```python
from build123d import *

# Parameters (mm, degrees)
SKETCH2_W           = 219.075
SKETCH2_H           = 241.3
BOSS_EXTRUDE1_DEPTH = 3.175
SKETCH3_W           = 3.175
SKETCH3_H           = 76.2
SKETCH3_W_2         = 76.2
SKETCH3_H_2         = 3.175
CUT_EXTRUDE1_DEPTH  = 4.175
SKETCH4_W           = 12.7
SKETCH4_H           = 20.32
SKETCH4_H_2         = 12.7
CUT_EXTRUDE2_DEPTH  = 4.175


with BuildPart() as part:
    # Sketch2 → Boss-Extrude1 (new body)
    with BuildSketch(Plane(origin=(0, 0, 0), x_dir=(1, 0, 0), z_dir=(0, 1, 0))):
        with Locations((109.5375, 120.65)):
            Rectangle(SKETCH2_W, SKETCH2_H)
    extrude(amount=BOSS_EXTRUDE1_DEPTH)

    # Sketch3 → Cut-Extrude1 (cut, through all)
    with BuildSketch(Plane(origin=(0, 3.175, 0), x_dir=(1, 0, 0), z_dir=(0, 1, 0))):
        with Locations((1.5875, 120.65)):
            Rectangle(SKETCH3_W, SKETCH3_H)
        with Locations((217.4875, 120.65)):
            Rectangle(SKETCH3_W, SKETCH3_H)
        with Locations((109.5375, 239.7125)):
            Rectangle(SKETCH3_W_2, SKETCH3_H_2)
        with Locations((109.5375, 1.5875)):
            Rectangle(SKETCH3_W_2, SKETCH3_H_2)
    extrude(amount=-CUT_EXTRUDE1_DEPTH, mode=Mode.SUBTRACT)

    # Sketch4 → Cut-Extrude2 (cut, through all)
    with BuildSketch(Plane(origin=(0, 3.175, 0), x_dir=(1, 0, 0), z_dir=(0, 1, 0))):
        with Locations((6.35, 60.96)):
            Rectangle(SKETCH4_W, SKETCH4_H)
        with Locations((6.35, 234.95)):
            Rectangle(SKETCH4_W, SKETCH4_H_2)
    extrude(amount=-CUT_EXTRUDE2_DEPTH, mode=Mode.SUBTRACT)


solid = part.part
```
The listing builds one solid part. Answer for the finished solid, in the listing's coordinates (mm). Give positions to 0.01 mm unless a question says otherwise; leave off trailing zeros. Order: outer loops, then holes, each group sorted by start corner. A loop starts at its lowest first (then second) coordinate and runs counter-clockwise, first axis right, second up.
Item 1: Find the intervals of material crossed by probe 1 along Z at (x, y) = (147, 0.75) (3 decimals); probe 2 along X at (y, z) = (1.4, -65) (3 decimals); probe 3 along X at (y, z) = (2.8, -152.5) (3 decimals), in increasing order.
From the geometry:
probe 1: z = -238.125 to -3.175
probe 2: x = 12.7 to 219.075
probe 3: x = 3.175 to 215.9
Item 2: Given pin 1 Ø1 at (y, z) = (1.5, -104.5) entering from -X (3 decimals); pin 2 Ø1 at (x, y) = (7, 2) entering from -Z; pin 3 Ø1 at (y, z) = (2, -240) entering from -X, each flat-ended and moving along its own axis, determine where each tip first touches the part or whether it passes through.
From the geometry:
pin 1: stops at x = 3.175
pin 2: stops at z = -228.6
pin 3: stops at x = 12.7
Item 3: The part is cut by section C-C, the plane x = 144. Give the vertices of the cut face in (y, z) (3 decimals), and give its area (3 significant figures).
From the geometry:
outline: (0, -238.125) - (3.175, -238.125) - (3.175, -3.175) - (0, -3.175) - close
area: 746 mm2
Item 4: The part is cut by section B-B, the plane z = -101. Give the vertices of the cut face in (x, y) (3 decimals), and give its area (3 significant figures).
From the geometry:
outline: (3.175, 0) - (215.9, 0) - (215.9, 3.175) - (3.175, 3.175) - close
area: 675 mm2
